Work out the finished part from the listing and answer in its coordinate system (mm). Give positions to 0.01 mm unless a question says otherwise; leave off trailing zeros. Order: outer loops, then holes, each group sorted by start corner. A loop starts at its lowest first (then second) coordinate and runs counter-clockwise, first axis right, second up. Notation, with made-up numbers: (72.5, 37.25) - (129.5, 37.25) arc R17 cw to (129.5, 42.25) - close; hole circle Ø7 at (24.5, -4.5). An arc over 180 degrees is marked (long way). Put each result on its own line as item: value.
Solid Edge part; units mm, degrees
sketch "Sketch1" plane through (0, 0, 0) normal (0, -1, 0) x (1, 0, 0)
  line L0 (-2.5, -1) -> (2.5, -1)
  line L1 (2.5, -1) -> (2.5, 1)
  line L2 (2.5, 1) -> (-2.5, 1)
  line L3 (-2.5, 1) -> (-2.5, -1)
extrude "Protrusion1" add sketch "Sketch1" along normal mid plane 35
fillet "Round_2" radius 2.5 4 edges at (-2.5, -17.5, 0) (2.5, -17.5, 0) (2.5, 17.5, 0) (-2.5, 17.5, 0)
hole "Hole_2" at (0, -15, 1) direction (0, 0, -1) diameter 2.6 end through all
hole "Hole1" at (0, 15, 1) direction (0, 0, -1) diameter 2.6 end through all
properties material "ABS Plastic, high impact"
(1) Section A-A, the plane z = -0.6 is taken. Count the separate pieces of the cut face and the enclosed holes in it, then the cut area to 3 significant figures.
Geometry check:
separate pieces: 1
enclosed holes: 2
area: 159 mm²
(2) Section B-B, the plane y = -14 is taken. Write down the section's boundary in (x, z), then the cut area to 3 significant figures.
Geometry check:
outline: (-2.5, -1) - (-0.83, -1) - (-0.83, 1) - (-2.5, 1) - close; (0.83, -1) - (2.5, -1) - (2.5, 1) - (0.83, 1) - close
area: 6.68 mm²
(3) Section C-C, the plane x = 1.6 is taken. Write down the section's boundary in (y, z).
Geometry check:
outline: (-16.92, -1) - (16.92, -1) - (16.92, 1) - (-16.92, 1) - close
(4) Straight lines are drawn through the part: line 1 (Y direction, x = 0, z = 0.2); line 2 (X direction, y = -15, z = 0.25); line 3 (Y direction, x = -0.85, z = 0.9). For each, find the intervals that lie inside material, in ascending order.
Geometry check:
line 1: y = -17.5 to -16.3, -13.7 to 13.7, 16.3 to 17.5
line 2: x = -2.5 to -1.3, 1.3 to 2.5
line 3: y = -17.35 to -15.98, -14.02 to 14.02, 15.98 to 17.35
(5) Determine the mould class of faces 1 (the face through (-1.748, -16.787, -0.014)), 2 (the face through (0, 0, -1)), 3 (the face through (0.06, -13.7, 0.01)) for opening direction X: pulls with the +X half, pulls with the -X half, needs draft (parallel to the pull), parting line crosses it, or undercut.
Geometry check:
face 1: pulls with the -X half
face 2: needs draft
face 3: undercut
(6) Section D-D, the plane x = -2 is taken. Write down the section's boundary in (y, z).
Geometry check:
outline: (-16.5, -1) - (16.5, -1) - (16.5, 1) - (-16.5, 1) - close
